Autodesk Inventor part; units mm, degrees
ref_plane "YZ Plane" through (0, 0, 0) normal (1, 0, 0) x (0, 1, 0)
ref_plane "XZ Plane" through (0, 0, 0) normal (0, 1, 0) x (-1, 0, 0)
ref_plane "XY Plane" through (0, 0, 0) normal (0, 0, 1) x (1, 0, 0)
sketch "Sketch1" plane through (0, 0, 0) normal (1, 0, 0) x (0, 1, 0)
  line L0 (57.5224, -43.6936) -> (57.5224, -57.6636)
  line L1 (57.5224, -57.6636) -> (39.4884, -57.6636)
  line L2 (39.4884, -57.6636) -> (39.4884, -43.6936)
  arc A0 (57.5224, -43.6936) -> (49.0054, -40.5737) centre (48.5054, -55.1236) ccw
  line L3 (67.5554, -43.7679) -> (67.5554, -94.5433)
  line L4 (29.4554, -43.7679) -> (29.4554, -94.5433)
  arc A1 (67.5554, -43.7679) -> (49.0054, -32.9515) centre (48.5054, -55.1236) ccw
  arc A2 (67.5554, -94.5433) -> (29.4554, -94.5433) centre (48.5054, -117.7186) ccw
  line L5 (60.5196, -70.9986) -> (60.5196, -67.8236)
  line L6 (55.5412, -67.8236) -> (55.5412, -70.9986)
  arc A3 (60.5196, -67.8236) -> (55.5412, -67.8236) centre (58.0304, -67.8236) ccw
  arc A4 (55.5412, -70.9986) -> (60.5196, -70.9986) centre (58.0304, -70.9986) ccw
  arc A5 (60.5196, -80.5236) -> (55.5412, -80.5236) centre (58.0304, -80.5236) ccw
  line L7 (60.5196, -83.6986) -> (60.5196, -80.5236)
  arc A6 (55.5412, -83.6986) -> (60.5196, -83.6986) centre (58.0304, -83.6986) ccw
  line L8 (55.5412, -80.5236) -> (55.5412, -83.6986)
  arc A7 (41.4696, -67.8236) -> (36.4912, -67.8236) centre (38.9804, -67.8236) ccw
  line L9 (41.4696, -70.9986) -> (41.4696, -67.8236)
  arc A8 (36.4912, -70.9986) -> (41.4696, -70.9986) centre (38.9804, -70.9986) ccw
  line L10 (36.4912, -67.8236) -> (36.4912, -70.9986)
  arc A9 (41.4696, -80.5236) -> (36.4912, -80.5236) centre (38.9804, -80.5236) ccw
  line L11 (41.4696, -83.6986) -> (41.4696, -80.5236)
  arc A10 (36.4912, -83.6986) -> (41.4696, -83.6986) centre (38.9804, -83.6986) ccw
  line L12 (36.4912, -80.5236) -> (36.4912, -83.6986)
  line L13 (48.5054, -117.7186) -> (48.5054, -32.9436) construction
  line L14 (57.5224, -50.6786) -> (39.4884, -50.6786) construction
  line L15 (48.0054, -40.5737) -> (48.0054, -32.9515)
  line L16 (49.0054, -32.9515) -> (49.0054, -40.5737)
  arc A11 (49.0054, -32.9515) -> (48.0054, -32.9515) centre (48.5054, -55.1236) ccw construction
  arc A12 (48.0054, -32.9515) -> (29.4554, -43.7679) centre (48.5054, -55.1236) ccw
  arc A13 (48.0054, -40.5737) -> (39.4884, -43.6936) centre (48.5054, -55.1236) ccw
  arc A14 (49.0054, -40.5737) -> (48.0054, -40.5737) centre (48.5054, -55.1236) ccw construction
  point P0 (0, 0)
  point P1 (48.5054, -40.5636)
  point P2 (48.5054, -50.6786)
  dimension "d0" = 13.97
  dimension "d1" = 18.034
  dimension "d2" = 2.54
  dimension "d4" = 30
  dimension "d8" = 4.9784
  dimension "d9" = 2.4892
  dimension "d17" = 3.175
  dimension "d20" = 12.7
  dimension "d23" = 19.05
  dimension "d26" = 38.1
  dimension "d30" = 10.16
  dimension "d31" = 7.62
  dimension "d32" = 67.04
  dimension "d33" = 1
extrude "Extrusion1" add sketch "Sketch1" along normal blind 12.7
sketch "Sketch2" plane through (12.7, 0, 0) normal (1, 0, 0) x (0, 0, -1)
  arc A0 (94.5433, 67.5554) -> (94.5433, 29.4554) centre (117.7186, 48.5054) ccw
  line L0 (90.8936, 61.9374) -> (64.8078, 61.9374)
  line L1 (62.3186, 59.4482) -> (62.3186, 37.5626)
  line L2 (64.8078, 35.0734) -> (90.8936, 35.0734)
  line L3 (87.7186, 48.5054) -> (62.3186, 48.5054) construction
  arc A1 (64.8078, 61.9374) -> (62.3186, 59.4482) centre (64.8078, 59.4482) ccw
  arc A2 (62.3186, 37.5626) -> (64.8078, 35.0734) centre (64.8078, 37.5626) ccw
  point P0 (0, 0)
  point P1 (62.3186, 61.9374)
  dimension "d37" = 25.4
  dimension "d38" = 28.575
  dimension "d39" = 2.4892
extrude "Extrusion2" cut sketch "Sketch2" against normal blind 6.35
properties part number "motormount2"
The model under review builds one solid part; all positions refer to its coordinate system, in mm. A direction names the side the tool comes from. Coordinates: 2 decimals unless noted, no trailing zeros. Write each loop counter-clockwise with the first axis right and the second up, starting at its lowest first coordinate (ties: lowest second). Pieces come first, ordered by that corner, then holes. Notation, with made-up numbers: (88.5, 27.25) - (95.5, 27.25) arc R19 cw to (95.5, 34.25) - close; hole circle Ø1 at (86.25, -37). An arc over 180 degrees is marked (long way). Answer as a JSON object with one key per item and string values. Group by question number.
1. Mouldability with a two-part tool opening along Z and no side actions: class faces 4 (the face through (6.261, 59.541, -35.886)), 5 (the face through (3, 60.52, -82)), 6 (the face through (0, 48, -63)) as pulls with the +Z half, pulls with the -Z half, needs draft (parallel to the pull), parting line crosses it, or undercut.
2. Add section C-C (z = -47.5). Give the boundary of the cut face in (x, y).
3. Add section B-B (x = 3). Give the boundary of the cut face in (y, z), plus the area to 3 significant figures.
4. Clearance check with flat-ended pins moving along their axes: pin 1 Ø1.9 at (x, y) = (10.5, 53.5) entering from -Z; pin 2 Ø1 at (x, y) = (4, 53) entering from +Z; pin 3 Ø8 at (y, z) = (43, -71) entering from +X. State where each tip first meets the part, or that it passes through.
5. Add section A-A (z = -81.5). Give the boundary of the cut face in (x, y), plus the area to 3 significant figures.
6. Machinability: for faces 1 (the face through (3.131, 39.035, -86.187)), 2 (the face through (10, 49, -62.319)), 3 (the face through (6, 29.455, -69)), which of the approach directions +Z, -Z, +X, -X, +Y, -Y give a long, thin tool a straight path to every point of the face, cutting with its end or side? Answer none if there is none.
7. To check wall thickness, follow probe 1 along Y at (x, z) = (3.5, -82); probe 2 along Y at (x, z) = (9.75, -85.5); probe 3 along Y at (x, z) = (2.75, -53). State the ranges of each line that lie inside material, in increasing order.
8. Add section D-D (y = 46). Give the boundary of the cut face in (x, z).
Findings:
{
 "1": {"face 4": "pulls with the +Z half", "face 5": "undercut", "face 6": "needs draft"},
 "2": {"outline": "(0, 29.46) - (12.7, 29.46) - (12.7, 39.49) - (0, 39.49) - close; (0, 57.52) - (12.7, 57.52) - (12.7, 67.56) - (0, 67.56) - close"},
 "3": {"outline": "(29.46, -94.54) arc R30 cw to (67.56, -94.54) - (67.56, -43.77) arc R22.18 ccw to (49.01, -32.95) - (49.01, -40.57) arc R14.56 cw to (57.52, -43.69) - (57.52, -57.66) - (39.49, -57.66) - (39.49, -43.69) arc R14.56 cw to (48.01, -40.57) - (48.01, -32.95) arc R22.18 ccw to (29.46, -43.77) - close; hole (36.49, -83.7) arc R2.49 ccw to (41.47, -83.7) - (41.47, -80.52) arc R2.49 ccw to (36.49, -80.52) - close; hole (36.49, -71) arc R2.49 ccw to (41.47, -71) - (41.47, -67.82) arc R2.49 ccw to (36.49, -67.82) - close; hole (55.54, -83.7) arc R2.49 ccw to (60.52, -83.7) - (60.52, -80.52) arc R2.49 ccw to (55.54, -80.52) - close; hole (55.54, -71) arc R2.49 ccw to (60.52, -71) - (60.52, -67.82) arc R2.49 ccw to (55.54, -67.82) - close", "area": "1,610 mm²"},
 "4": {"pin 1": "z = -62.32", "pin 2": "z = -33.31", "pin 3": "x = 6.35"},
 "5": {"outline": "(0, 29.46) - (12.7, 29.46) - (12.7, 35.07) - (6.35, 35.07) - (6.35, 36.49) - (0, 36.49) - close; (0, 41.47) - (6.35, 41.47) - (6.35, 55.54) - (0, 55.54) - close; (0, 60.52) - (6.35, 60.52) - (6.35, 61.94) - (12.7, 61.94) - (12.7, 67.56) - (0, 67.56) - close", "area": "250 mm²"},
 "6": {"face 1": "+X, -X", "face 2": "-Z, +X", "face 3": "+Z, -Z, +X, -X, -Y"},
 "7": {"probe 1": "29.46 to 36.49, 41.47 to 55.54, 60.52 to 67.56", "probe 2": "29.46 to 35.07, 61.94 to 67.56", "probe 3": "29.46 to 39.49, 57.52 to 67.56"},
 "8": {"outline": "(0, -87.82) - (6.35, -87.82) - (6.35, -62.32) - (12.7, -62.32) - (12.7, -57.66) - (0, -57.66) - close; (0, -40.78) - (12.7, -40.78) - (12.7, -33.09) - (0, -33.09) - close"}
}
